from build123d import *

# Parameters (mm, degrees)
F0_W     = 27.94
F0_H     = 25.4
F0_R     = 4.064
F1_DEPTH = 10.16
F2_W     = 20.066
F2_H     = 6.604
F3_DEPTH = 14.224
F4_R     = 1.905
F5_DEPTH = 3.0226
F6_DEPTH = 17.78


with BuildPart() as f1:
    # F0 (on Top) → F1 (new body)
    with BuildSketch(Plane.XY):
        with Locations((-11.43, 0)):
            Rectangle(F0_W, F0_H)
        with Locations((-5.588, 0)):
            Circle(F0_R, mode=Mode.SUBTRACT)
    extrude(amount=F1_DEPTH)

    # F2 (on face) → F3 (cut)
    with BuildSketch(Plane(origin=(-25.4, 0, 0), x_dir=(0, -1, 0), z_dir=(-1, 0, 0))):
        with Locations((0, 5.08)):
            Rectangle(F2_W, F2_H)
    extrude(amount=-F3_DEPTH, mode=Mode.SUBTRACT)

    # F4 (on face) → F5 (cut)
    with BuildSketch(Plane.XZ.offset(12.7)):
        with Locations((-13.081, 5.08)):
            Circle(F4_R)
    extrude(amount=-F5_DEPTH, mode=Mode.SUBTRACT)

    # F0 (on Top) → F6 (join)
    with BuildSketch(Plane.XY):
        with Locations((-11.43, 0)):
            Rectangle(F0_W, F0_H)
        with Locations((-5.588, 0)):
            Circle(F0_R, mode=Mode.SUBTRACT)
    extrude(amount=-F6_DEPTH)


solid = f1.part
Input: part model. Units: mm. Frame: model coordinates. A direction names the side the tool comes from. Round coordinates to 2 decimals unless told otherwise and drop trailing zeros. Order: outer loops, then holes, each group sorted by start corner. A loop starts at its lowest first (then second) coordinate and runs counter-clockwise, first axis right, second up.
1. Cut plane D-D, the plane y = 6.5. Output: boundary loops of the cut face in (x, z).
The answers:
outline: (-25.4, -17.78) - (2.54, -17.78) - (2.54, 10.16) - (-25.4, 10.16) - (-25.4, 8.38) - (-11.18, 8.38) - (-11.18, 1.78) - (-25.4, 1.78) - close
2. Cut plane A-A, the plane y = 0. Output: boundary loops of the cut face in (x, z), then the cut area to 3 significant figures.
The answers:
outline: (-25.4, -17.78) - (-9.65, -17.78) - (-9.65, 10.16) - (-25.4, 10.16) - (-25.4, 8.38) - (-11.18, 8.38) - (-11.18, 1.78) - (-25.4, 1.78) - close; (-1.52, -17.78) - (2.54, -17.78) - (2.54, 10.16) - (-1.52, 10.16) - close
area: 460 mm2
3. Pin query (flat end, axial travel): P1, Ø6.5, axis at x = -5.588, y = 0, coming from the +Z side. Return the tip coordinate at first contact, or that it passes through.
The answers:
P1: passes through
4. Material intervals for line 1 (Z direction, x = -18.75, y = -9); line 2 (Y direction, x = -6.5, z = -5.5); line 3 (X direction, y = -3.5, z = -6.25), sorted ascending.
The answers:
line 1: z = -17.78 to 1.78, 8.38 to 10.16
line 2: y = -12.7 to -3.96, 3.96 to 12.7
line 3: x = -25.4 to -7.65, -3.52 to 2.54
5. Set-up query: faces 4 (the face through (-18, 0, 1.778)), 5 (the face through (-12, 12.7, -4)), 6 (the face through (-11.3, -11.4, 4.4)). Return all of +Z, -Z, +X, -X, +Y, -Y with unobstructed straight access to the full face (end or side cutting, diameter ignored); none if empty.
The answers:
face 4: -X
face 5: +Z, -Z, +X, -X, +Y
face 6: -Y
6. Cut plane C-C, the plane z = 0.5. Output: boundary loops of the cut face in (x, y).
The answers:
outline: (-25.4, -12.7) - (2.54, -12.7) - (2.54, 12.7) - (-25.4, 12.7) - close; hole circle Ø8.13 at (-5.59, 0)
7. Mould query, pull axis Z, two halves, no side actions, for faces 1 (the face through (-18, -10.033, 5)), 2 (the face through (-12, 0, -17.78)), 3 (the face through (-1.834, -1.557, -4.006)). Classes: released by +Z, released by -Z, zero draft, split by the parting line, or undercut.
The answers:
face 1: undercut
face 2: released by -Z
face 3: zero draft
8. Cut plane B-B, the plane x = -17. Output: boundary loops of the cut face in (y, z).
The answers:
outline: (-12.7, -17.78) - (12.7, -17.78) - (12.7, 10.16) - (-12.7, 10.16) - close; hole (-10.03, 1.78) - (10.03, 1.78) - (10.03, 8.38) - (-10.03, 8.38) - close
